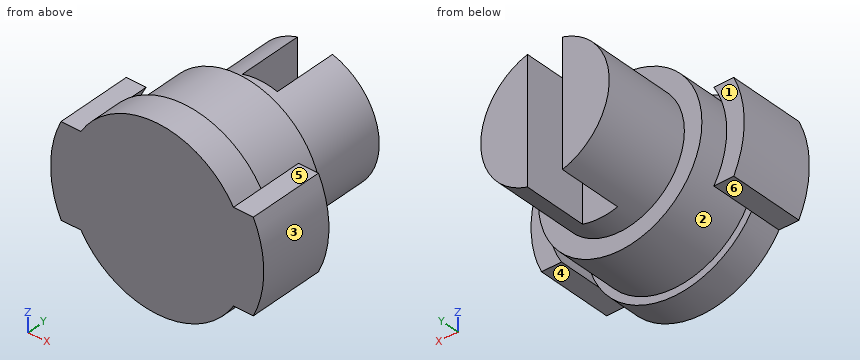
Autodesk Inventor part; units mm, degrees
ref_plane "YZ Plane" through (0, 0, 0) normal (1, 0, 0) x (0, 1, 0)
ref_plane "XZ Plane" through (0, 0, 0) normal (0, 1, 0) x (-1, 0, 0)
ref_plane "XY Plane" through (0, 0, 0) normal (0, 0, 1) x (1, 0, 0)
sketch "Sketch1" plane through (0, 0, 0) normal (0, 1, 0) x (-1, 0, 0)
  circle A0 centre (0, 0) radius 14
  dimension "d0" = 28
extrude "Extrusion1" add sketch "Sketch1" along normal blind 16.5
sketch "Sketch2" plane through (0, 16.5, 0) normal (0, 1, 0) x (1, 0, 0)
  circle A0 centre (0, 0) radius 11
  dimension "d3" = 22
extrude "Extrusion2" add sketch "Sketch2" along normal blind 15
sketch "Sketch3" plane through (0, 31.5, 0) normal (0, 1, 0) x (1, 0, 0)
  line L0 (-3, -11) -> (3, -11)
  line L1 (3, -11) -> (3, 11)
  line L2 (3, 11) -> (-3, 11)
  line L3 (-3, 11) -> (-3, -11)
  line L4 (-3, -11) -> (3, 11) construction
  line L5 (3, -11) -> (-3, 11) construction
  circle A0 centre (0, 0) radius 11
  point P0 (3, -10.583)
  point P1 (3, 10.583)
  point P2 (-3, 10.583)
  point P3 (-3, -10.583)
  dimension "d6" = 6
  dimension "d7" = 0
extrude "Extrusion3" cut sketch "Sketch3" against normal blind 11 contours A0 L3 L1
sketch "Sketch4" plane through (0, 0, 0) normal (0, -1, 0) x (1, 0, 0)
  circle A0 centre (0, 0) radius 15.25
  dimension "d10" = 30.5
extrude "Extrusion4" add sketch "Sketch4" against normal blind 5.5
sketch "Sketch5" plane through (0, 0, 0) normal (0, -1, 0) x (1, 0, 0)
  line L0 (-16.4635, -7.875) -> (16.4635, -7.875)
  line L1 (16.4635, 7.875) -> (-16.4635, 7.875)
  circle A0 centre (0, 0) radius 15.25
  arc A1 (-16.4635, 7.875) -> (-16.4635, -7.875) centre (0, 0) ccw
  arc A2 (16.4635, -7.875) -> (16.4635, 7.875) centre (0, 0) ccw
  point P0 (-13.0594, -7.875)
  point P1 (-13.0594, 7.875)
  point P2 (13.0594, 7.875)
  point P3 (13.0594, -7.875)
  dimension "d15" = 15.75
  dimension "d16" = 7.875
  dimension "d17" = 18.25
  dimension "d18" = 18.25
  dimension "d19" = 0
extrude "Extrusion5" add sketch "Sketch5" against normal blind 13 contours A1 L1 A0 L0 | A0 L1 A2 L0
properties part number "Light Water Sensor"
CAD build for the part. Positions are in the model's coordinates, mm. Face numbers are marked on the shaded views. A direction names the side the tool comes from. Round coordinates to 2 decimals unless told otherwise and drop trailing zeros. Write each loop counter-clockwise with the first axis right and the second up, starting at its lowest first coordinate (ties: lowest second). Pieces come first, ordered by that corner, then holes. Notation, with made-up numbers: (-5.75, 28) - (1.25, 28) arc R30 ccw to (1.25, 51) - close; hole circle Ø8 at (55.25, -32.5). An arc over 180 degrees is marked (long way). Write item = value, one per line. Start each with the question number.
Q1. Band-saw the part on D-D (y = 29.5). Give the cut face in (x, z), then the cut area to 3 significant figures.
Q2. Mould opens along Z. For the marked faces 1, 2 and 3 say: pulls with the +Z half, pulls with the -Z half, needs draft (parallel to the pull), parting line crosses it, or undercut.
Q3. Band-saw the part on C-C (x = 0). Give the cut face in (y, z).
Q4. Which spindle directions (+Z, -Z, +X, -X, +Y, -Y) get a long thin tool onto all of the face, cutting with end or side? Do the marked faces 4, 5 and 6. Say none if no direction does.
Q5. Probe L1, parallel to X at y = 8.5, z = 0.5; L2, parallel to Z at x = 0.5, y = 4.5; L3, parallel to Y at x = -12.5, z = -8. List the from-to ranges inside material, lowest first. Write a range as from..to.
Q6. Band-saw the part on A-A (z = 0). Give the cut face in (x, y).
Q7. Drop flat-ended pins along their axis: pin 1 (2.5 mm diameter, centred on x = -14.5, z = 1.5, fed in from +Y); pin 2 (1 mm diameter, centred on x = 4.5, y = 15, fed in from +Z); pin 3 (1.5 mm diameter, centred on x = 14, y = 7.5, fed in from +Z) (3 decimals). Give the stop position or say it passes through.
Answers below:
q1.outline = (-3, -10.58) - (-3, 10.58) arc R11 ccw to start; (3, -10.58) arc R11 ccw to (3, 10.58) - close
q1.area = 250 mm2
q2.face_1 = needs draft
q2.face_2 = undercut
q2.face_3 = parting line crosses it
q3.outline = (0, -15.25) - (5.5, -15.25) - (5.5, -14) - (16.5, -14) - (16.5, -11) - (20.5, -11) - (20.5, 11) - (16.5, 11) - (16.5, 14) - (5.5, 14) - (5.5, 15.25) - (0, 15.25) - close
q4.face_4 = -Z, +X, +Y, -Y
q4.face_5 = +Z, +X, +Y, -Y
q4.face_6 = -Z, -X, +Y, -Y
q5.L1 = -18.24..-15.24, -13.99..13.99, 15.24..18.24
q5.L2 = -15.24..15.24
q5.L3 = 0..5.5
q6.outline = (-18.25, 0) - (18.25, 0) - (18.25, 13) - (15.25, 13) - (15.25, 5.5) - (14, 5.5) - (14, 16.5) - (11, 16.5) - (11, 31.5) - (3, 31.5) - (3, 20.5) - (-3, 20.5) - (-3, 31.5) - (-11, 31.5) - (-11, 16.5) - (-14, 16.5) - (-14, 5.5) - (-15.25, 5.5) - (-15.25, 13) - (-18.25, 13) - close
q7.pin_1 = 16.5
q7.pin_2 = 13.42
q7.pin_3 = 7.875
